Build history of the part. All positions in model axes, mm. Face numbers are marked on the shaded views. A direction names the side the tool comes from. Give positions to 0.01 mm unless a question says otherwise; leave off trailing zeros. Order: outer loops, then holes, each group sorted by start corner. A loop starts at its lowest first (then second) coordinate and runs counter-clockwise, first axis right, second up. Notation, with made-up numbers: (-14, -4) - (-7, -4) arc R17 ccw to (-7, 13) - close; hole circle Ø2 at (32, 0). An arc over 180 degrees is marked (long way). Write each question's results on one line, items separated by ' | '. Start each with the question number.
1) Drill centre lines: line 1 along Y through (x, z) = (1, -4); line 2 along X through (y, z) = (47.5, 15). Where is each one in solid material? Low to high. Write a range as from..to.
2) Tool access for the marked faces 1, 2, 3 and 4: list every direction of +Z, -Z, +X, -X, +Y, -Y with a clear straight run to the whole face (end or side of a thin tool).
3) Two-plate mould, pull along Z, no slides. Class the marked faces 5, 6 and 7: +Z half, -Z half, draft (parallel to the pull), parting line (faces both ways), or undercut.
4) Cut at B-B on y = 45. List the corners of the cut face in (x, z), plus the area to 3 significant figures.
5) Cut at C-C on z = 45. List the corners of the cut face in (x, y).
6) Cut at D-D on y = 10.5. State how many separate pieces and enclosed holes the cut face has, plus the area to 3 significant figures.
7) Cut at A-A on z = -4. List the corners of the cut face in (x, y), plus the area to 3 significant figures.
8) Drop flat-ended pins along their axis: pin 1 Ø11.5 at (x, y) = (12, 31) entering from +Z; pin 2 Ø5.5 at (x, z) = (14, 15) entering from +Y; pin 3 Ø1.1 at (x, z) = (21.5, 39.5) entering from -Y; pin 4 Ø0.8 at (y, z) = (71.5, 1.5) entering from -X. Give the stop position or say it passes through.
Autodesk Fusion 360 part; units mm, degrees
sketch "Sketch1" plane through (0, 0, 0) normal (0, 1, 0) x (1, 0, 0)
  line L0 (0, 0) -> (41, 0)
  line L1 (41, 0) -> (41, -41)
  line L2 (41, -41) -> (0, -41)
  line L3 (0, -41) -> (0, 0)
  line L4 (1, -1) -> (40, -1)
  line L5 (40, -1) -> (40, -40)
  line L6 (40, -40) -> (1, -40)
  line L7 (1, -40) -> (1, -1)
  line L8 (20, -40) -> (20, -1)
  line L9 (21, -40) -> (21, -1)
  line L10 (1, -21) -> (20, -21)
  line L11 (1, -20) -> (20, -20)
  line L12 (21, -21) -> (40, -21)
  line L13 (21, -20) -> (40, -20)
  dimension "d1" = 41
  dimension "d2" = 41
  dimension "d3" = 39
  dimension "d4" = 1
  dimension "d5" = 1
  dimension "d6" = 19
  dimension "d7" = 19
  dimension "d8" = 1
  dimension "d9" = 1
  dimension "d10" = 19
  dimension "d11" = 19
extrude "Extrude1" add sketch "Sketch1" along normal blind 68 contours L4 L6 L8 L9 | L7 L8 L10 L11 | L5 L9 L12 L13
extrude "Extrude2" add sketch "Sketch1" along normal blind 72
extrude "Extrude3" add sketch "Sketch1" along normal blind 2 contours L4 L7 L8 L11 | L4 L5 L9 L13 | L6 L7 L8 L10 | L5 L6 L9 L12
ref_plane "WorkPlane1" through (18, 37, 20.5) normal (1, 0, 0) x (0, 0, -1)
sketch "Sketch6" plane through (18, 0, 0) normal (1, 0, 0) x (0, 1, 0)
  line L0 (72, 40) -> (70.5, 40)
  line L1 (70.5, 40) -> (70.5, 39)
  line L2 (70.5, 39) -> (72, 40)
  line L3 (72, 1) -> (70.5, 1)
  line L4 (70.5, 1) -> (70.5, 2)
  line L5 (70.5, 2) -> (72, 1)
extrude "Extrude4" add sketch "Sketch6" along normal blind 5
fillet "Fillet1" radius 1 1 edges at (41, 36, 41)
fillet "Fillet2" radius 1 1 edges at (0, 36, 41)
fillet "Fillet3" radius 1 5 edges at (41, 0, 20) (40.7071, 0, 40.7071) (20.5, 0, 41) (0.2929, 0, 40.7071) (0, 0, 20)
fillet "Fillet4" radius 1 5 edges at (41, 36.5, 0) (40.7071, 0.2929, 0) (20.5, 0, 0) (0.2929, 0.2929, 0) (0, 36.5, 0)
sketch "Sketch8" plane through (0, 0, 0) normal (-1, 0, 0) x (0, -1, 0)
  line L0 (-72, 1) -> (-1, 1)
  line L1 (-1, 1) -> (-1, 40)
  line L2 (-1, 40) -> (-72, 40)
  line L3 (-72, 40) -> (-72, 1)
  line L4 (-72, 1) -> (0, 1)
  line L5 (0, 1) -> (0, -7.5)
  line L6 (0, -7.5) -> (-72, -7.5)
  line L7 (-72, -7.5) -> (-72, 1)
  line L8 (0, 40) -> (-72, 40)
  line L9 (-72, 40) -> (-72, 48.5)
  line L10 (-72, 48.5) -> (0, 48.5)
  line L11 (0, 48.5) -> (0, 40)
  circle A0 centre (-68.5, 45) radius 2.5
  circle A1 centre (-10.5, 45) radius 2.5
  circle A2 centre (-68.5, -4) radius 2.5
  circle A3 centre (-10.5, -4) radius 2.5
  dimension "d41" = 8.5
  dimension "d42" = 8.5
  dimension "d44" = 5
  dimension "d45" = 5
  dimension "d46" = 5
  dimension "d47" = 5
  dimension "d48" = 3.5
  dimension "d49" = 3.5
  dimension "d50" = 3.5
  dimension "d51" = 3.5
  dimension "d52" = 3.5
  dimension "d53" = 3.5
  dimension "d54" = 58
  dimension "d55" = 58
extrude "Extrude5" add sketch "Sketch8" along normal blind 0 and the other way blind 2 contours L0 L4 L5 L6 L7 | L2 L8 L9 L10 L11 | A0 | A1 | A2 | A3
extrude "Extrude6" add sketch "Sketch8" along normal blind 3.5 contours A0 | A1 | A2 | A3
hole "Hole1" at (0, 68.5, 45) direction (1, 0, 0) diameter 2.076 depth 6 tip angle 180
hole "Hole2" at (0, 68.5, 45) direction (-1, 0, 0) diameter 2.076 depth 2.5 tip angle 180
hole "Hole3" at (0, 10.5, 45) direction (1, 0, 0) diameter 2.076 depth 11 tip angle 180
hole "Hole4" at (0, 10.5, 45) direction (-1, 0, 0) diameter 2.076 depth 11 tip angle 180
hole "Hole5" at (0, 10.5, -4) direction (1, 0, 0) diameter 2.076 depth 9 tip angle 180
hole "Hole6" at (0, 10.5, -4) direction (-1, 0, 0) diameter 2.076 depth 9 tip angle 180
hole "Hole7" at (0, 68.5, -4) direction (1, 0, 0) diameter 2.076 depth 9 tip angle 180
hole "Hole8" at (0, 68.5, -4) direction (-1, 0, 0) diameter 2.076 depth 9 tip angle 180
hole "Hole9" at (0, 68.5, 45) at (0, 10.5, 45) at (0, 10.5, -4) at (0, 68.5, -4) direction (1, 0, 0) diameter 2.529 end through all
hole "Hole10" at (0, 10.5, 45) at (0, 68.5, 45) at (0, 10.5, -4) at (0, 68.5, -4) direction (1, 0, 0) diameter 2.529 depth 6 tip angle 180
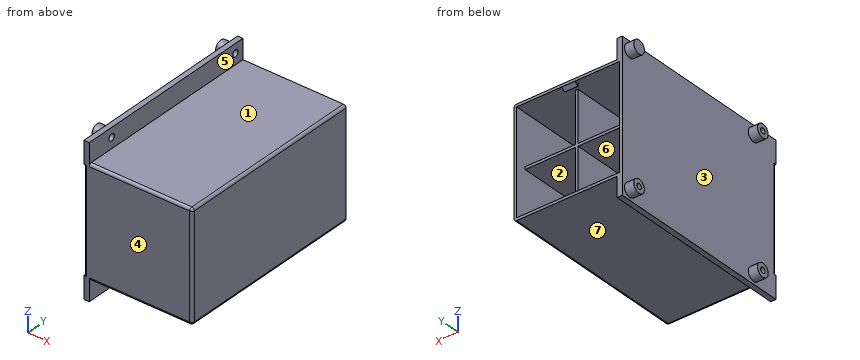
Results:
1) line 1: 0..9.24, 11.76..67.24, 69.76..72 | line 2: 0..1, 20..21, 40..41
2) face 1: +Z, +X, +Y, -Y | face 2: +Y | face 3: -X | face 4: +Z, -Z, +X, -X, -Y
3) face 5: draft | face 6: undercut | face 7: -Z half
4) outline: (0, -7.5) - (2, -7.5) - (2, 0) - (40, 0) arc R1 ccw to (41, 1) - (41, 40) arc R1 ccw to (40, 41) - (2, 41) - (2, 48.5) - (0, 48.5) - close; hole (1, 1) - (20, 1) - (20, 20) - (1, 20) - close; hole (1, 21) - (20, 21) - (20, 40) - (1, 40) - close; hole (21, 1) - (40, 1) - (40, 20) - (21, 20) - close; hole (21, 21) - (40, 21) - (40, 40) - (21, 40) - close | area: 267 mm^2
5) outline: (-3.5, 8) - (0, 8) - (0, 0) - (2, 0) - (2, 9.24) - (0, 9.24) - (0, 9.46) - (-3.5, 9.46) - close; (-3.5, 11.54) - (0, 11.54) - (0, 11.76) - (2, 11.76) - (2, 67.24) - (0, 67.24) - (0, 67.46) - (-2.5, 67.46) - (-2.5, 69.54) - (0, 69.54) - (0, 69.76) - (2, 69.76) - (2, 72) - (0, 72) - (0, 71) - (-3.5, 71) - (-3.5, 66) - (0, 66) - (0, 13) - (-3.5, 13) - close
6) separate pieces: 3 | enclosed holes: 4 | area: 277 mm^2
7) outline: (-3.5, 8) - (0, 8) - (0, 0) - (2, 0) - (2, 9.24) - (0, 9.24) - (0, 9.46) - (-3.5, 9.46) - close; (-3.5, 11.54) - (0, 11.54) - (0, 11.76) - (2, 11.76) - (2, 67.24) - (0, 67.24) - (0, 67.46) - (-3.5, 67.46) - (-3.5, 66) - (0, 66) - (0, 13) - (-3.5, 13) - close; (-3.5, 69.54) - (0, 69.54) - (0, 69.76) - (2, 69.76) - (2, 72) - (0, 72) - (0, 71) - (-3.5, 71) - close | area: 154 mm^2
8) pin 1: z = 41 | pin 2: y = 2 | pin 3: y = 0 | pin 4: x = 0
